```python
from build123d import *

# Parameters (mm, degrees)
F0_W     = 101.6
F0_H     = 30.48
F1_DEPTH = 63.5
F2_T     = -2.54
F4_D     = 7.9375
F4_DEPTH = 12.7
F5_W     = 19.05
F5_H     = 9.525
F6_DEPTH = 25.4


with BuildPart() as f1:
    # F0 (on Front) → F1 (new body)
    with BuildSketch(Plane.XZ):
        with Locations((50.8, 15.24)):
            Rectangle(F0_W, F0_H)
    extrude(amount=F1_DEPTH)

    # F2
    f2_openings = [f1.faces().sort_by_distance(p)[0] for p in [
        (50.8, -31.75, 30.48),
    ]]
    offset(amount=F2_T, openings=f2_openings)

    # F4
    with Locations(Plane.YZ.offset(101.6)):
        with Locations((-12.34637, 12.614627)):
            Hole(F4_D / 2, depth=F4_DEPTH)

    # F5 (on face) → F6 (cut)
    with BuildSketch(Plane.YZ.offset(101.6)):
        with Locations((-42.752528, 14.270137)):
            Rectangle(F5_W, F5_H)
    extrude(amount=-F6_DEPTH, mode=Mode.SUBTRACT)


solid = f1.part
```
Model file for the job. Use its own axes, mm. A direction names the side the tool comes from. Round coordinates to 2 decimals unless told otherwise and drop trailing zeros. Loops run counter-clockwise (first coordinate to the right, second up) from the corner with the lowest first, then second, coordinate; pieces in that order, holes last. Notation, with made-up numbers: M -15,-32 L 38,-32 A23 ccw 38,-4 Z; hole C 60.25,35.25 d4. An arc over 180 degrees is marked long. Put each result on its own line as item: value. Start each with the question number.
Item 1: Cut at C-C (x = 74). List the corners of the cut face in (y, z).
Item 2: Mould opens along X. For faces 1 (the face through (50, -60.96, 17)), 2 (the face through (50, -63.5, 15)), 3 (the face through (2.54, -31, 16)), 4 (the face through (0, -31, 15)) say: released by +X, released by -X, zero draft, split by the parting line, or undercut.
Item 3: Cut at B-B (y = -36). List the corners of the cut face in (x, z), then the cut area to 3 significant figures.
Item 4: Drop flat-ended pins along their axis: P1, Ø1.5, axis at x = 15, z = 11, coming from the +Y side; P2, Ø1, axis at x = 10.5, y = -7, coming from the +Z side. Give the stop position or say it passes through.
Item 5: Cut at A-A (z = 27.5). List the corners of the cut face in (x, y).
Item 6: Cut at D-D (z = 11). List the corners of the cut face in (x, y), then the cut area to 3 significant figures.
Item 7: Drill centre lines: line 1 along Y through (x, z) = (46, 3.5); line 2 along X through (y, z) = (-39, 22.5); line 3 along Z through (x, y) = (38.5, -19). Where is each one in solid material? Low to high.
Item 8: 3-axis set-ups, long thin cutter, end or side, ignore diameter. For faces 5 (the face through (101.6, -31, 15)), 6 (the face through (50, -31, 2.54)), 7 (the face through (100, -52.278, 14)): which of +Z, -Z, +X, -X, +Y, -Y reach the whole face in a straight line?
Answer block:
1. outline: M -63.5,0 L 0,0 L 0,30.48 L -2.54,30.48 L -2.54,2.54 L -60.96,2.54 L -60.96,30.48 L -63.5,30.48 Z
2. face 1: undercut
2. face 2: zero draft
2. face 3: undercut
2. face 4: released by -X
3. outline: M 0,0 L 101.6,0 L 101.6,9.51 L 99.06,9.51 L 99.06,2.54 L 2.54,2.54 L 2.54,30.48 L 0,30.48 Z; M 99.06,19.03 L 101.6,19.03 L 101.6,30.48 L 99.06,30.48 Z
3. area: 376 mm2
4. P1: y = 0
4. P2: z = 2.54
5. outline: M 0,-63.5 L 101.6,-63.5 L 101.6,0 L 0,0 Z; hole M 2.54,-60.96 L 99.06,-60.96 L 99.06,-2.54 L 2.54,-2.54 Z
6. outline: M 0,-63.5 L 101.6,-63.5 L 101.6,-52.28 L 99.06,-52.28 L 99.06,-60.96 L 2.54,-60.96 L 2.54,-2.54 L 99.06,-2.54 L 99.06,-8.72 L 101.6,-8.72 L 101.6,0 L 0,0 Z; M 99.06,-33.23 L 101.6,-33.23 L 101.6,-15.97 L 99.06,-15.97 Z
6. area: 746 mm2
7. line 1: -63.5 to -60.96, -2.54 to 0
7. line 2: 0 to 2.54, 99.06 to 101.6
7. line 3: 0 to 2.54
8. face 5: +Z, -Z, +X, +Y, -Y
8. face 6: +Z
8. face 7: +X
